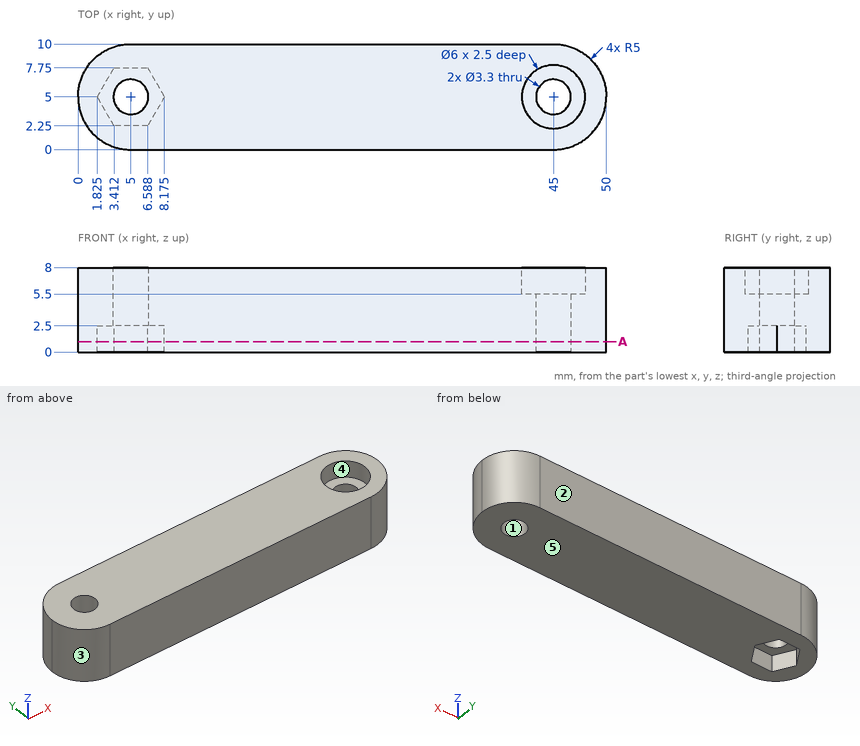
For this review, use the dimensioned drawing (mm, ordinates from the lowest corner) and the shaded views. A direction names the side the tool comes from. Round coordinates to 2 decimals unless told otherwise and drop trailing zeros. Answer in a Markdown table with one row per item.
Q1. Take a section at A-A, the plane z = 1. Count the separate pieces of the cut face and the enclosed holes in it, then the cut area to 3 significant figures.
The answers:
| item | result |
|---|---|
| separate pieces | 1 |
| enclosed holes | 2 |
| area | 444 mm² |
Q2. Clearance check with flat-ended pins moving along their axes: pin 1 Ø5.5 at (x, y) = (45, 5) entering from +Z; pin 2 Ø3 at (y, z) = (1.5, 3.5) entering from -X. State where each tip first meets the part, or that it passes through.
The answers:
| item | result |
|---|---|
| pin 1 | z = 5.5 |
| pin 2 | x = 0.42 |
Q3. Draft analysis for pull direction Y (two halves, no side actions). For the marked faces 1, 2 and 3, state which applies: +Y half, -Y half, draft (parallel to the pull), parting line (faces both ways), or undercut.
The answers:
| item | result |
|---|---|
| face 1 | undercut |
| face 2 | +Y half |
| face 3 | -Y half |
Q4. For the marked faces 4 and 5, list the 3-axis set-ups (+Z, -Z, +X, -X, +Y, -Y) from which the entire face can be reached by the end or side of a thin tool; tool diameter is ignored.
The answers:
| item | result |
|---|---|
| face 4 | +Z |
| face 5 | -Z, +X, -X, +Y, -Y |
Q5. To check wall thickness, follow L1, parallel to X at y = 4.5, z = 7 (1 decimal); L2, parallel to Y at x = 5, z = 5.8; L3, parallel to X at y = 4.5, z = 3 (1 decimal). State the ranges of each line that lie inside material, in increasing order. Write a range as [from, to].
The answers:
| item | result |
|---|---|
| L1 | [0, 3.4], [6.6, 42], [48, 50] |
| L2 | [0, 3.35], [6.65, 10] |
| L3 | [0, 3.4], [6.6, 43.4], [46.6, 50] |
